Source: CAD feature listing. Evaluate the final solid. Frame: model axes, mm. A direction names the side the tool comes from. Give positions to 0.01 mm unless a question says otherwise; leave off trailing zeros. Loops run counter-clockwise (first coordinate to the right, second up) from the corner with the lowest first, then second, coordinate; pieces in that order, holes last. Notation, with made-up numbers: (29.5, -30.75) -> (71.5, -30.75) arc R17 ccw to (71.5, -21.75) -> close; hole circle Ø4 at (-38.75, 9). An arc over 180 degrees is marked (long way). Return JSON: item names as keys, results as strings. Group by question number.
(1) Cut plane B-B on y = 4.25. Return loops of the section in (x, z), then the cut area to 3 significant figures.
(2) Cut plane D-D on z = 0.5. Give the number of separate pieces and of enclosed holes in the cut face, then the cut area to 3 significant figures.
(3) Cut plane C-C on y = -0.5. Return loops of the section in (x, z).
(4) Ray query, line 1 (X direction, y = -4.5, z = 0); line 2 (Z direction, x = 1.5, y = -1.25) (3 decimals); line 3 (X direction, y = -2.5, z = -2). Return the intervals inside material, ascending. Write a range as from..to.
(5) Draft query along X for faces 1 (the face through (-2.4, 0.1, -3.2)), 2 (the face through (-2.636, -0.111, -0.585)), 3 (the face through (-1, 7.95, 3)). Return one class per face: released by +X, released by -X, zero draft, split by the parting line, or undercut.
(6) Cut plane A-A on x = 0. Return loops of the section in (y, z), then the cut area to 3 significant figures.
(7) Pin query (flat end, axial travel): pin 1 (2 mm diameter, centred on y = -4, z = 3, fed in from +X); pin 2 (2 mm diameter, centred on x = -3, y = 1, fed in from -Z). Return the tip coordinate at first contact, or that it passes through.
(8) Access query for faces 4 (the face through (-0.601, 6.158, 2.892)), 5 (the face through (-1, -7.95, 3)). Directions: +Z, -Z, +X, -X, +Y, -Y. A direction counts if a zero-diameter tool reaches every point of the face in a straight line with its end or side. Return the directions, or none.
```python
from build123d import *

# Parameters (mm, degrees)
SKETCH1_R           = 4
SKETCH1_R_2         = 2.7
BOSS_EXTRUDE1_DEPTH = 7.95
SKETCH2_R           = 2
CUT_EXTRUDE1_DEPTH  = 10.757176846
CIRPATTERN1_COUNT   = 2
CIRPATTERN1_ANGLE   = 105


with BuildPart() as part:
    # Sketch1 → Boss-Extrude1 (new, symmetric)
    with BuildSketch(Plane(origin=(0, 0, 0), x_dir=(1, 0, 0), z_dir=(0, 1, 0))):
        with Locations(Location((0, 0, 0), (0, 0, 270))):
            Circle(SKETCH1_R)
        with Locations(Location((0, 0, 0), (0, 0, 270))):
            Circle(SKETCH1_R_2, mode=Mode.SUBTRACT)
    extrude(amount=BOSS_EXTRUDE1_DEPTH, both=True)

    # Sketch2 → Cut-Extrude1 (cut, through all)
    with BuildSketch(Plane.XY):
        with Locations(Location((0, 4.25, 0), (0, 0, 90.000000002))):
            Circle(SKETCH2_R)
    cut_extrude1 = extrude(amount=CUT_EXTRUDE1_DEPTH, mode=Mode.SUBTRACT)

    # CirPattern1: Cut-Extrude1 ×2 about axis
    cirpattern1_axis = Axis((0, 7.95, 0), (0, 1, 0))
    for i in range(1, CIRPATTERN1_COUNT):
        add(cut_extrude1.rotate(cirpattern1_axis, i * CIRPATTERN1_ANGLE / (CIRPATTERN1_COUNT - 1)), mode=Mode.SUBTRACT)


solid = part.part
```
Answers:
{
 "1": {"outline": "(-2, 1.81) -> (-2, 3.46) arc R4 ccw (long way) to (2.83, -2.83) -> (1.23, -2.4) arc R2.7 cw to start; (2, 1.81) arc R2.7 cw to (2.27, 1.46) -> (3.86, 1.04) arc R4 ccw to (2, 3.46) -> close", "area": "16.2 mm²"},
 "2": {"separate pieces": "3", "enclosed holes": "0", "area": "37.9 mm²"},
 "3": {"outline": "circle Ø8 at (0, 0); hole circle Ø5.4 at (0, 0)"},
 "4": {"line 1": "-4..-2.7, 2.7..4", "line 2": "-3.708..-2.245, 2.245..3.708", "line 3": "-3.46..-1.81, 1.81..3.46"},
 "5": {"face 1": "split by the parting line", "face 2": "undercut", "face 3": "zero draft"},
 "6": {"outline": "(-7.95, -4) -> (7.95, -4) -> (7.95, -2.7) -> (-7.95, -2.7) -> close; (-7.95, 2.7) -> (2.25, 2.7) -> (2.25, 4) -> (-7.95, 4) -> close; (6.25, 2.7) -> (7.95, 2.7) -> (7.95, 4) -> (6.25, 4) -> close", "area": "36.1 mm²"},
 "7": {"pin 1": "x = 3.46", "pin 2": "z = -3.46"},
 "8": {"face 4": "+Z", "face 5": "+Z, -Z, +X, -X, -Y"}
}
